Can you work these out from the drawing? Everything is in mm from the part's minimum corner. A direction names the side the tool comes from. Coordinates: 2 decimals unless noted, no trailing zeros. Loops run counter-clockwise (first coordinate to the right, second up) from the corner with the lowest first, then second, coordinate; pieces in that order, holes last. Notation, with made-up numbers: (-3.5, 58.25) - (43.5, 58.25) arc R22 cw to (43.5, 65.25) - close; hole circle Ø8 at (-4, -11). An arc over 180 degrees is marked (long way). Put each result on its own line as item: value. Start each with the question number.
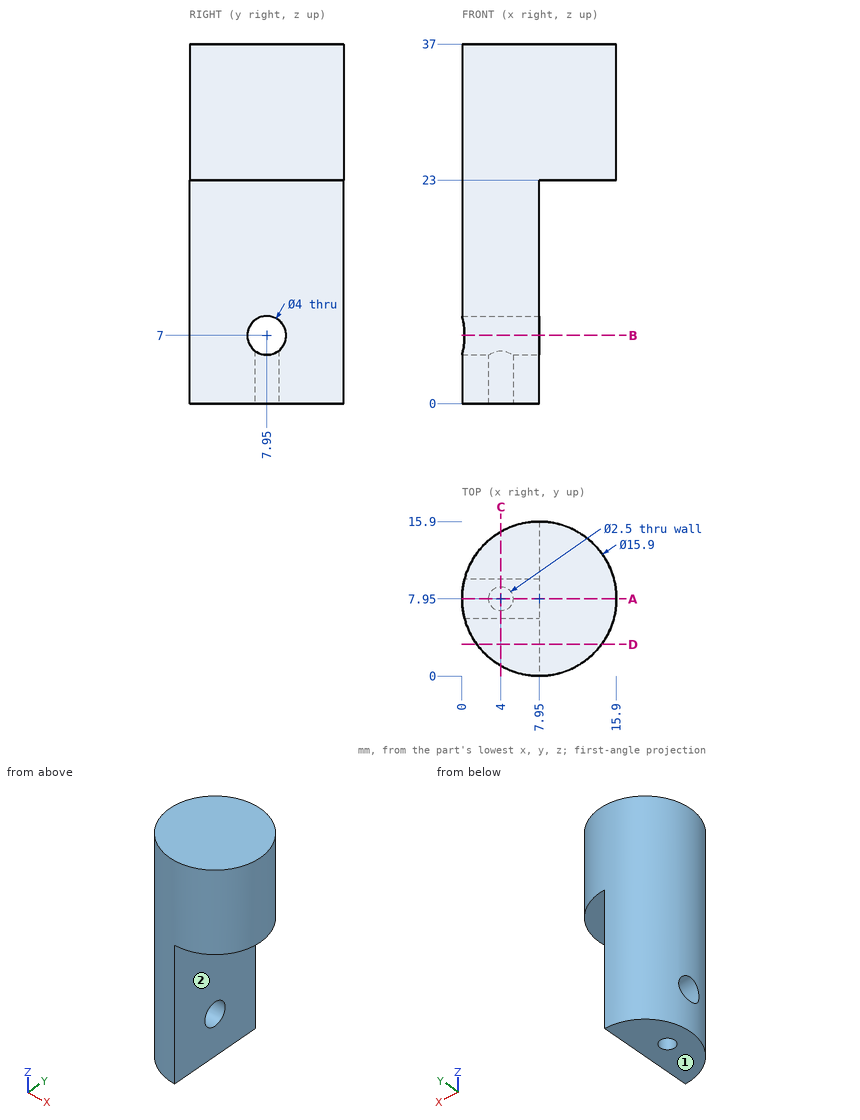
(1) Which directions (+Z, -Z, +X, -X, +Y, -Y) give clear straight access to the entire face, cutting with the end or side of a thin tool? Please do the marked faces 1 and 2.
(2) I want a section at C-C on x = 4. List the corners of the cut face in (y, z) for me, and give its area (3 significant figures).
(3) I want a section at D-D on y = 3.25. List the corners of the cut face in (x, z) for me, and give its area (3 significant figures).
(4) I want a section at B-B on z = 7. List the corners of the cut face in (x, y) for me.
(5) I need wall thicknesses on L1, parallel to Z at x = 9.75, y = 10.25; L2, parallel to Z at x = 3.75, y = 7.95; L3, parallel to Z at x = 6.75, y = 7.95. Which ranges of each line are inside material? Lowest first, please. Write a range as [from, to].
(6) For pin 1 Ø8 at (y, z) = (13.5, 25) entering from +X; pin 2 Ø2 at (y, z) = (12, 21) entering from +X; pin 3 Ø3 at (x, z) = (11.5, 31.5) entering from +Y; pin 4 Ø3.5 at (y, z) = (7.95, 7) entering from -X, each with a flat end and sliding along its axis, tell me the tip position at first contact or that it passes through.
(7) I want a section at A-A on y = 7.95. List the corners of the cut face in (x, z) for me.
Answer sheet:
1. face 1: -Z, +X, -X, +Y, -Y
1. face 2: -Z, +X, +Y, -Y
2. outline: (1.05, 0) - (6.7, 0) - (6.7, 5.44) arc R2 cw (long way) to (9.2, 5.44) - (9.2, 0) - (14.85, 0) - (14.85, 37) - (1.05, 37) - close
2. area: 485 mm^2
3. outline: (1.54, 0) - (7.95, 0) - (7.95, 23) - (14.36, 23) - (14.36, 37) - (1.54, 37) - close
3. area: 327 mm^2
4. outline: (0.26, 5.95) arc R7.95 ccw to (7.95, 0) - (7.95, 5.95) - close; (0.26, 9.95) - (7.95, 9.95) - (7.95, 15.9) arc R7.95 ccw to start
5. L1: z = [23, 37]
5. L2: z = [9, 37]
5. L3: z = [0, 5], [9, 37]
6. pin 1: stops at x = 15.75
6. pin 2: stops at x = 7.95
6. pin 3: stops at y = 15.63
6. pin 4: passes through
7. outline: (0, 0) - (2.75, 0) - (2.75, 5) - (0, 5) - close; (0, 9) - (7.95, 9) - (7.95, 23) - (15.9, 23) - (15.9, 37) - (0, 37) - close; (5.25, 0) - (7.95, 0) - (7.95, 5) - (5.25, 5) - close
